Autodesk Inventor part; units mm, degrees
ref_plane "YZ Plane" through (0, 0, 0) normal (1, 0, 0) x (0, 1, 0)
ref_plane "XZ Plane" through (0, 0, 0) normal (0, 1, 0) x (-1, 0, 0)
ref_plane "XY Plane" through (0, 0, 0) normal (0, 0, 1) x (1, 0, 0)
sketch "Sketch1" plane through (0, 0, 0) normal (0, 1, 0) x (-1, 0, 0)
  line L0 (0, 0) -> (0, 6)
  line L1 (-3, 0) -> (-3, 6)
  line L2 (-3, 6) -> (-4, 6)
  line L3 (-4, 6) -> (-4, 1)
  line L4 (-4, 1) -> (-6, 1)
  line L5 (-6, 1) -> (-6, 0)
  line L6 (-6, 0) -> (-3, 0)
  dimension "InsideDiameter" = 6
  dimension "OuterDiameter" = 8
  dimension "FlangeDiameter" = 12
  dimension "FlangeThickness" = 1
  dimension "Length" = 5
revolve "Revolution1" add sketch "Sketch1" angle 360 about axis through (0, 0, 0) along (0, 0, 1)
chamfer "Chamfer1" distance 0.3 angle 30 1 edges at (-4, 0, 6) measured on face at (3.9482, -0.6416, 4.3333)
fillet "Fillet1" radius 0.5 1 edges at (-4, 0, 1)
properties part number "GFM-0608-06" material "Acetal Resin, Black"
Model file for the job. Use its own axes, mm. Round coordinates to 2 decimals unless told otherwise and drop trailing zeros. Write each loop counter-clockwise with the first axis right and the second up, starting at its lowest first coordinate (ties: lowest second). Pieces come first, ordered by that corner, then holes. Notation, with made-up numbers: M 40.5,28 L 47.5,28 A23 ccw 47.5,56 Z; hole C 86.25,-19.75 d2. An arc over 180 degrees is marked long. Put each result on its own line as item: value.
Item 1: Cut at C-C (z = 0.8). List the corners of the cut face in (x, y), and give its area (3 significant figures).
Responses:
outline: C 0,0 d12; hole C 0,0 d6
area: 84.8 mm²
Item 2: Cut at A-A (x = 0). List the corners of the cut face in (y, z), and give its area (3 significant figures).
Responses:
outline: M -6,0 L -3,0 L -3,6 L -3.83,6 L -4,5.7 L -4,1.5 A0.5 cw -4.5,1 L -6,1 Z; M 3,0 L 6,0 L 6,1 L 4.5,1 A0.5 cw 4,1.5 L 4,5.7 L 3.83,6 L 3,6 Z
area: 16.1 mm²
Item 3: Probe L1, parallel to Y at x = 0, z = 3.4; L2, parallel to Z at x = -3.5, y = -2.75; L3, parallel to X at y = -2.75, z = 1.55. List the from-to ranges inside material, lowest first. Write a range as from..to.
Responses:
L1: -4..-3, 3..4
L2: 0..1
L3: -2.9..-1.2, 1.2..2.9
Item 4: Mould opens along X. For faces 1 (the cylindrical face through (-3, 0, 3)), 2 (the cylindrical face through (-0.867, 3.905, 3.571)), 3 (the flat face through (-1.4, 4.5, 1)) say: +X half, -X half, draft (parallel to the pull), parting line (faces both ways), or undercut.
Responses:
face 1: undercut
face 2: parting line
face 3: draft
Item 5: Flat gauge pins, fed straight in: P1, Ø5.5, axis at x = 0, y = 0, coming from the -Z side; P2, Ø1.5, axis at y = -3.5, z = 4, coming from the -X side; P3, Ø2, axis at y = 4.5, z = 5.5, coming from the +X side; P4, Ø1, axis at x = 2.5, z = 4, coming from the +Y side. Where does each tip first touch, or does it go through?
Responses:
P1: through
P2: x = -2.9
P3: x = 1.94
P4: y = 3.46
Item 6: Cut at D-D (z = 5.4). List the corners of the cut face in (x, y).
Responses:
outline: C 0,0 d8; hole C 0,0 d6
